```python
from build123d import *

# Parameters (mm, degrees)
F0_R     = 11.9868187185
F0_R_2   = 6.9041541384
F1_DEPTH = 24.384
F0_W     = 70.5220922828
F0_H     = 42.4831844866
F2_DEPTH = 25.4


# Not quite as in the source:
# - the program builds the solid bodies; features that only make, move or delete a surface that nothing else refers to are left out


with BuildPart() as f1:
    # F0 (on Front) → F1 (new body)
    with BuildSketch(Plane.XZ):
        Circle(F0_R)
        Circle(F0_R_2, mode=Mode.SUBTRACT)
    extrude(amount=F1_DEPTH)

    # F0 (on Front) → F2 (join)
    with BuildSketch(Plane.XZ):
        Rectangle(F0_W, F0_H)
        Circle(F0_R, mode=Mode.SUBTRACT)
    extrude(amount=F2_DEPTH)


solid = f1.part
```
Source: CAD feature listing. Evaluate the final solid. Frame: model axes, mm. A direction names the side the tool comes from. Give positions to 0.01 mm unless a question says otherwise; leave off trailing zeros. Write each loop counter-clockwise with the first axis right and the second up, starting at its lowest first coordinate (ties: lowest second). Pieces come first, ordered by that corner, then holes. Notation, with made-up numbers: (57, 80.5) - (90, 80.5) arc R16 ccw to (90, 99.5) - close; hole circle Ø6 at (88, 89). An arc over 180 degrees is marked (long way). One line per item, written item: value. Start each with the question number.
Q1. Section query A-A, the plane x = 0. Return the cut outline in (y, z).
Q2. Section query B-B, the plane z = 0. Return the cut outline in (x, y), then the cut area to 3 significant figures.
Q3. Set-up query: faces 4 (the face through (5, -24.384, -5)), 5 (the face through (-6.897, -12.021, 0.304)). Return all of +Z, -Z, +X, -X, +Y, -Y with unobstructed straight access to the full face (end or side cutting, diameter ignored); none if empty.
Q4. Draft query along X for faces 1 (the face through (11.433, -24.885, 3.601)), 2 (the face through (-8, -25.4, 10)), 3 (the face through (-35.261, -13, 0)). Return one class per face: +X half, -X half, draft (parallel to the pull), parting line (faces both ways), or undercut.
Q5. Section query D-D, the plane x = 8.5. Return the cut outline in (y, z).
Q6. First-contact query: pin 1 Ø4 at (x, z) = (7, 6) entering from -Y. Flat tip, straight axial feed; report the tip coordinate or a pass-through.
Q7. Section query C-C, the plane y = -8.25. Return the cut outline in (x, z).
Q8. Material intervals for probe 1 along Z at (x, y) = (0, -24.95); probe 2 along Z at (x, y) = (0, -17.75); probe 3 along X at (y, z) = (-2.25, -2.5), sorted ascending. Write a range as from..to.
Answer:
1. outline: (-25.4, -21.24) - (0, -21.24) - (0, -6.9) - (-24.38, -6.9) - (-24.38, -11.99) - (-25.4, -11.99) - close; (-25.4, 11.99) - (-24.38, 11.99) - (-24.38, 6.9) - (0, 6.9) - (0, 21.24) - (-25.4, 21.24) - close
2. outline: (-35.26, -25.4) - (-11.99, -25.4) - (-11.99, -24.38) - (-6.9, -24.38) - (-6.9, 0) - (-35.26, 0) - close; (6.9, -24.38) - (11.99, -24.38) - (11.99, -25.4) - (35.26, -25.4) - (35.26, 0) - (6.9, 0) - close
2. area: 1,430 mm2
3. face 4: -Y
3. face 5: +Y, -Y
4. face 1: undercut
4. face 2: draft
4. face 3: -X half
5. outline: (-25.4, -21.24) - (0, -21.24) - (0, 21.24) - (-25.4, 21.24) - (-25.4, 8.45) - (-24.38, 8.45) - (-24.38, -8.45) - (-25.4, -8.45) - close
6. pin 1: stops at y = -24.38
7. outline: (-35.26, -21.24) - (35.26, -21.24) - (35.26, 21.24) - (-35.26, 21.24) - close; hole circle Ø13.81 at (0, 0)
8. probe 1: z = -21.24..-11.99, 11.99..21.24
8. probe 2: z = -21.24..-6.9, 6.9..21.24
8. probe 3: x = -35.26..-6.44, 6.44..35.26
